from build123d import *

# Parameters (mm, degrees)
SKETCH1_R           = 4
BOSS_EXTRUDE1_DEPTH = 1


with BuildPart() as part:
    # Sketch1 → Boss-Extrude1 (new, symmetric)
    with BuildSketch(Plane(origin=(0, 0, 0), x_dir=(1, 0, 0), z_dir=(0, 1, 0))):
        with BuildLine():
            Line((-181.921418525, 102.72297888), (-187.187405589, 105.763297929))
            ThreePointArc((-187.187405589, 105.763297929), (-215, 0), (-187.187405589, -105.763297929))
            Line((-187.187405589, -105.763297929), (-181.921418525, -102.72297888))
            Line((-181.921418525, -102.72297888), (-179.921418525, -106.187080495))
            Line((-179.921418525, -106.187080495), (-185.187405589, -109.227399544))
            ThreePointArc((-185.187405589, -109.227399544), (-107.5, -186.195461814), (-2, -214.990697473))
            Line((-2, -214.990697473), (-2, -208.910059376))
            Line((-2, -208.910059376), (2, -208.910059376))
            Line((2, -208.910059376), (2, -214.990697473))
            ThreePointArc((2, -214.990697473), (107.5, -186.195461814), (185.187405589, -109.227399544))
            Line((185.187405589, -109.227399544), (179.921418525, -106.187080495))
            Line((179.921418525, -106.187080495), (181.921418525, -102.72297888))
            Line((181.921418525, -102.72297888), (187.187405589, -105.763297929))
            ThreePointArc((187.187405589, -105.763297929), (215, 0), (187.187405589, 105.763297929))
            Line((187.187405589, 105.763297929), (181.921418525, 102.72297888))
            Line((181.921418525, 102.72297888), (179.921418525, 106.187080495))
            Line((179.921418525, 106.187080495), (185.187405589, 109.227399544))
            ThreePointArc((185.187405589, 109.227399544), (107.5, 186.195461814), (2, 214.990697473))
            Line((2, 214.990697473), (2, 208.910059376))
            Line((2, 208.910059376), (-2, 208.910059376))
            Line((-2, 208.910059376), (-2, 214.990697473))
            ThreePointArc((-2, 214.990697473), (-107.5, 186.195461814), (-185.187405589, 109.227399544))
            Line((-185.187405589, 109.227399544), (-179.921418525, 106.187080495))
            Line((-179.921418525, 106.187080495), (-181.921418525, 102.72297888))
        make_face()
        with Locations(Location((-15, -129.131715701, 0), (0, 0, 270))):
            Circle(SKETCH1_R, mode=Mode.SUBTRACT)
        with Locations(Location((-119.331346232, -51.575476794, 0), (0, 0, 270))):
            Circle(SKETCH1_R, mode=Mode.SUBTRACT)
        with Locations(Location((-104.331346232, -77.556238907, 0), (0, 0, 270))):
            Circle(SKETCH1_R, mode=Mode.SUBTRACT)
        with Locations(Location((-12.5, -79.017403146, 0), (0, 0, 270))):
            Circle(SKETCH1_R, mode=Mode.SUBTRACT)
        with Locations(Location((-62.181078466, -50.334019121, 0), (0, 0, 270))):
            Circle(SKETCH1_R, mode=Mode.SUBTRACT)
        with Locations(Location((-74.681078466, -28.683384026, 0), (0, 0, 270))):
            Circle(SKETCH1_R, mode=Mode.SUBTRACT)
        with Locations(Location((15, -129.131715701, 0), (0, 0, 270))):
            Circle(SKETCH1_R, mode=Mode.SUBTRACT)
        with Locations(Location((12.5, -79.017403146, 0), (0, 0, 270))):
            Circle(SKETCH1_R, mode=Mode.SUBTRACT)
        with Locations(Location((104.331346232, -77.556238907, 0), (0, 0, 270))):
            Circle(SKETCH1_R, mode=Mode.SUBTRACT)
        with BuildLine():
            Line((-10.609274752, 3.826177687), (-8.609274752, 7.290279302))
            Line((-8.609274752, 7.290279302), (-2.96077803, 4.029118199))
            ThreePointArc((-2.96077803, 4.029118199), (-2.491557477, 4.33499035), (-1.9910703, 4.586462587))
            Line((-1.9910703, 4.586462587), (-1.9910703, 11.100990294))
            Line((-1.9910703, 11.100990294), (2.0089297, 11.100990294))
            Line((2.0089297, 11.100990294), (2.0089297, 4.578668088))
            ThreePointArc((2.0089297, 4.578668088), (2.50843303, 4.325247245), (2.976457964, 4.017548754))
            Line((2.976457964, 4.017548754), (8.618204452, 7.274812608))
            Line((8.618204452, 7.274812608), (10.618204452, 3.810710993))
            Line((10.618204452, 3.810710993), (4.96970773, 0.549549889))
            ThreePointArc((4.96970773, 0.549549889), (4.999990507, -0.009743105), (4.967528264, -0.568913833))
            Line((4.967528264, -0.568913833), (10.609274752, -3.826177687))
            Line((10.609274752, -3.826177687), (8.609274752, -7.290279302))
            Line((8.609274752, -7.290279302), (2.96077803, -4.029118199))
            ThreePointArc((2.96077803, -4.029118199), (2.491557477, -4.33499035), (1.9910703, -4.586462587))
            Line((1.9910703, -4.586462587), (1.9910703, -11.100990294))
            Line((1.9910703, -11.100990294), (-2.0089297, -11.100990294))
            Line((-2.0089297, -11.100990294), (-2.0089297, -4.578668088))
            ThreePointArc((-2.0089297, -4.578668088), (-2.50843303, -4.325247245), (-2.976457964, -4.017548754))
            Line((-2.976457964, -4.017548754), (-8.618204452, -7.274812608))
            Line((-8.618204452, -7.274812608), (-10.618204452, -3.810710993))
            Line((-10.618204452, -3.810710993), (-4.96970773, -0.549549889))
            ThreePointArc((-4.96970773, -0.549549889), (-4.999990507, 0.009743105), (-4.967528264, 0.568913833))
            Line((-4.967528264, 0.568913833), (-10.609274752, 3.826177687))
        make_face(mode=Mode.SUBTRACT)
        with Locations(Location((62.181078466, -50.334019121, 0), (0, 0, 270))):
            Circle(SKETCH1_R, mode=Mode.SUBTRACT)
        with Locations(Location((74.681078466, -28.683384026, 0), (0, 0, 270))):
            Circle(SKETCH1_R, mode=Mode.SUBTRACT)
        with Locations(Location((119.331346232, -51.575476794, 0), (0, 0, 270))):
            Circle(SKETCH1_R, mode=Mode.SUBTRACT)
        with Locations(Location((-119.331346232, 51.575476794, 0), (0, 0, 270))):
            Circle(SKETCH1_R, mode=Mode.SUBTRACT)
        with Locations(Location((-74.681078466, 28.683384026, 0), (0, 0, 270))):
            Circle(SKETCH1_R, mode=Mode.SUBTRACT)
        with Locations(Location((-62.181078466, 50.334019121, 0), (0, 0, 270))):
            Circle(SKETCH1_R, mode=Mode.SUBTRACT)
        with Locations(Location((-104.331346232, 77.556238907, 0), (0, 0, 270))):
            Circle(SKETCH1_R, mode=Mode.SUBTRACT)
        with Locations(Location((-12.5, 79.017403146, 0), (0, 0, 270))):
            Circle(SKETCH1_R, mode=Mode.SUBTRACT)
        with Locations(Location((-15, 129.131715701, 0), (0, 0, 270))):
            Circle(SKETCH1_R, mode=Mode.SUBTRACT)
        with Locations(Location((74.681078466, 28.683384026, 0), (0, 0, 270))):
            Circle(SKETCH1_R, mode=Mode.SUBTRACT)
        with Locations(Location((62.181078466, 50.334019121, 0), (0, 0, 270))):
            Circle(SKETCH1_R, mode=Mode.SUBTRACT)
        with Locations(Location((12.5, 79.017403146, 0), (0, 0, 270))):
            Circle(SKETCH1_R, mode=Mode.SUBTRACT)
        with Locations(Location((104.331346232, 77.556238907, 0), (0, 0, 270))):
            Circle(SKETCH1_R, mode=Mode.SUBTRACT)
        with Locations(Location((119.331346232, 51.575476794, 0), (0, 0, 270))):
            Circle(SKETCH1_R, mode=Mode.SUBTRACT)
        with Locations(Location((15, 129.131715701, 0), (0, 0, 270))):
            Circle(SKETCH1_R, mode=Mode.SUBTRACT)
    extrude(amount=BOSS_EXTRUDE1_DEPTH, both=True)


solid = part.part
Input: part model. Units: mm. Frame: model coordinates. Give positions to 0.01 mm unless a question says otherwise; leave off trailing zeros. Order: outer loops, then holes, each group sorted by start corner. A loop starts at its lowest first (then second) coordinate and runs counter-clockwise, first axis right, second up. Notation, with made-up numbers: (34.5, -24.5) -> (59.5, -24.5) arc R30 ccw to (59.5, 5.5) -> close; hole circle Ø9 at (-35.5, -15.75). An arc over 180 degrees is marked (long way). Use one line per item in the form item = value.
1) Line query: probe 1 along X at (y, z) = (0.95, 50.5); probe 2 along Z at (x, y) = (-102, -0.05); probe 3 along X at (y, z) = (-0.5, -79). Output: solid intervals per line, ascending.
Response values:
probe_1 = -208.99 to -123.18, -115.48 to -66.18, -58.18 to 58.18, 66.18 to 115.48, 123.18 to 208.99
probe_2 = -189.26 to -80.81, -74.31 to 74.31, 80.81 to 189.26
probe_3 = -199.96 to -108.06, -100.6 to -16.5, -8.5 to 8.5, 16.5 to 100.6, 108.06 to 199.96
2) Section C-C, the plane z = -88. Return loops of the section in (x, y).
Response values:
outline = (-196.17, -1) -> (196.17, -1) -> (196.17, 1) -> (-196.17, 1) -> close
3) Section B-B, the plane x = 162. Return loops of the section in (y, z).
Response values:
outline = (-1, -141.35) -> (1, -141.35) -> (1, 141.35) -> (-1, 141.35) -> close
4) First-contact query: pin 1 Ø6.5 at (x, z) = (15, -129.13) entering from -Y; pin 2 Ø13 at (x, z) = (-119.33, 51.58) entering from -Y; pin 3 Ø0.6 at (y, z) = (0, -8.5) entering from +X. Flat tips, straight axial feed; report the tip coordinate or a pass-through.
Response values:
pin_1 = through
pin_2 = -1
pin_3 = 214.84
5) Section A-A, the plane y = -0.05. Count the separate pieces of the cut face and the enclosed holes in it, and give its area (3 significant figures).
Response values:
separate_pieces = 1
enclosed_holes = 25
area = 144,000 mm^2
